Input: dimensioned drawing with shaded views. Units: mm. Origin: part minimum x, y, z. Round coordinates to 2 decimals unless told otherwise and drop trailing zeros. Loops run counter-clockwise (first coordinate to the right, second up) from the corner with the lowest first, then second, coordinate; pieces in that order, holes last. Notation, with made-up numbers: M 81.5,7.25 L 135.5,7.25 A23 cw 135.5,46.25 Z; hole C 77.5,-19.5 d7. An arc over 180 degrees is marked long. Answer as a JSON object with one key per item and string values.
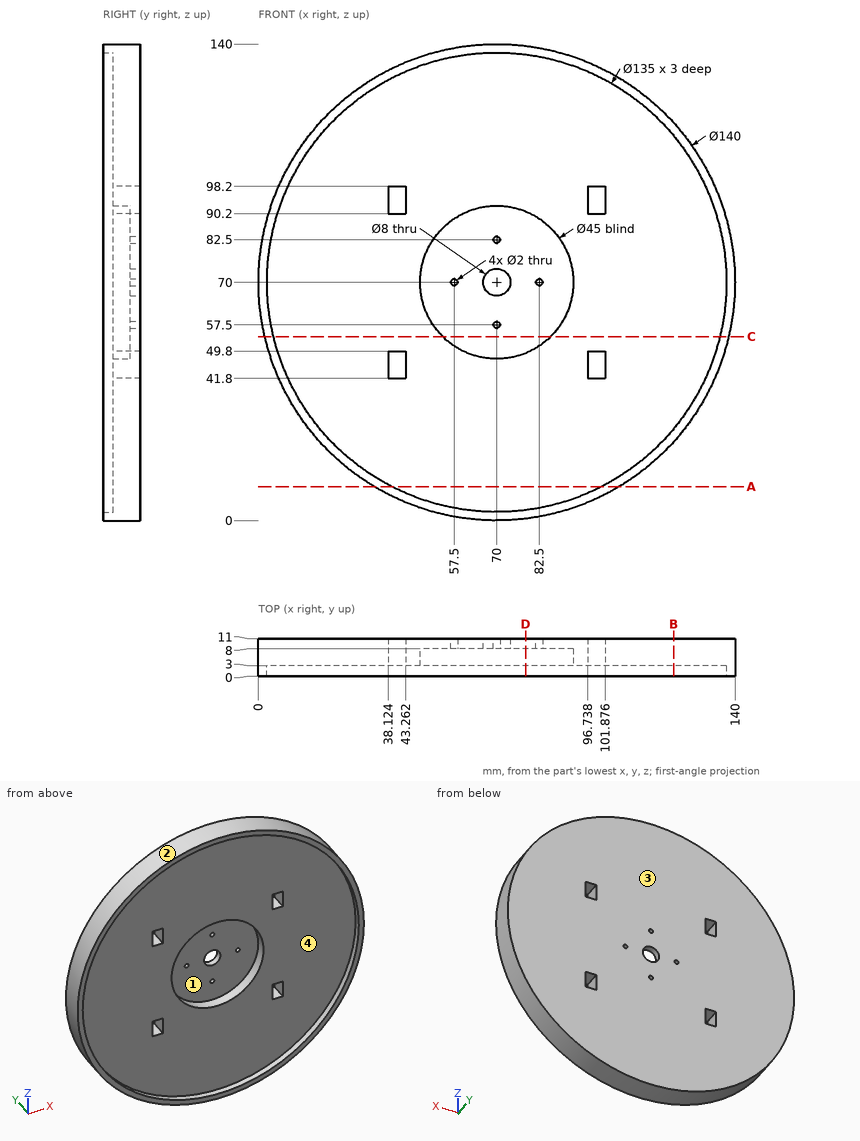
Item 1: Section B-B on x = 122. Return the cut outline in (y, z).
Answer sheet:
{"outline": "M 0,23.14 L 11,23.14 L 11,116.86 L 0,116.86 L 0,113.04 L 3,113.04 L 3,26.96 L 0,26.96 Z"}
Item 2: Section D-D on x = 78.5. Return the cut outline in (y, z).
Answer sheet:
{"outline": "M 0,0.52 L 11,0.52 L 11,139.48 L 0,139.48 L 0,136.96 L 3,136.96 L 3,90.83 L 8,90.83 L 8,49.17 L 3,49.17 L 3,3.04 L 0,3.04 Z"}
Item 3: Section A-A on z = 10. Return the cut outline in (x, y) (1 decimal), then the cut area to 3 significant figures.
Answer sheet:
{"outline": "M 33.9,0 L 39.1,0 L 39.1,3 L 100.9,3 L 100.9,0 L 106.1,0 L 106.1,11 L 33.9,11 Z", "area": "608 mm²"}
Item 4: Line query: probe 1 along X at (y, z) = (9.5, 70); probe 2 along Z at (x, y) = (97, 7.75); probe 3 along X at (y, z) = (6, 70). Output: solid intervals per line, ascending. Write a range as from..to.
Answer sheet:
{"probe 1": "x = 0..56.5, 58.5..66, 74..81.5, 83.5..140", "probe 2": "z = 5.42..41.8, 49.8..90.2, 98.2..134.58", "probe 3": "x = 0..47.5, 92.5..140"}
Item 5: Section C-C on z = 54. Return the cut outline in (x, y).
Answer sheet:
{"outline": "M 1.85,0 L 4.42,0 L 4.42,3 L 54.18,3 L 54.18,8 L 85.82,8 L 85.82,3 L 135.58,3 L 135.58,0 L 138.15,0 L 138.15,11 L 1.85,11 Z"}
Item 6: Contact query for flat-ended pins moving along their axis: pin 1 Ø2 at (x, z) = (122, 49.5) entering from -Y; pin 2 Ø2.5 at (x, y) = (40.5, 8) entering from +Z; pin 3 Ø1 at (y, z) = (6, 79.5) entering from -X. Output: stop coordinate, or through.
Answer sheet:
{"pin 1": "stops at y = 3", "pin 2": "stops at z = 134.05", "pin 3": "stops at x = 0.58"}
Item 7: Pull-direction query (X, two-part tool) for the marked faces 1, 2, 3 and 4; classes: pulls with the +X half, pulls with the -X half, needs draft (parallel to the pull), parting line crosses it, or undercut.
Answer sheet:
{"face 1": "undercut", "face 2": "parting line crosses it", "face 3": "needs draft", "face 4": "undercut"}
